Verification items for the finished model (mm, model axes). A direction names the side the tool comes from. Give positions to 0.01 mm unless a question says otherwise; leave off trailing zeros. Loops run counter-clockwise (first coordinate to the right, second up) from the corner with the lowest first, then second, coordinate; pieces in that order, holes last. Notation, with made-up numbers: (-28, 83.25) - (-15, 83.25) arc R21 ccw to (-15, 96.25) - close; hole circle Ø3 at (32, 19.25). An arc over 180 degrees is marked (long way). Answer in a Markdown table with one row per item.
```python
from build123d import *

# Parameters (mm, degrees)
SKETCH1_R               = 3.175
BOSS_EXTRUDE1_DEPTH     = 111.76
SKETCH2_R               = 2.667
BOSS_EXTRUDE2_DEPTH     = 0.762
SKETCH3_R               = 3.175
BOSS_EXTRUDE3_DEPTH     = 1.27
FILLET1_R               = 0.254
CUT_EXTRUDE1_DEPTH      = 114.880553719
CUT_EXTRUDE1_DEPTH_BACK = 114.880553719
SKETCH4_R               = 1.143


with BuildPart() as part:
    # Sketch1 → Boss-Extrude1 (new body)
    with BuildSketch(Plane(origin=(0, 0, 0), x_dir=(0, 0, -1), z_dir=(1, 0, 0))):
        Circle(SKETCH1_R)
    extrude(amount=-BOSS_EXTRUDE1_DEPTH)

    # Sketch2 → Boss-Extrude2 (add)
    with BuildSketch(Plane.ZY.offset(111.76)):
        with Locations(Location((0, 0, 0), (0, 0, 180))):
            Circle(SKETCH2_R)
    extrude(amount=BOSS_EXTRUDE2_DEPTH)

    # Sketch3 → Boss-Extrude3 (add)
    with BuildSketch(Plane.ZY.offset(112.522)):
        with Locations(Location((0, 0, 0), (0, 0, 180))):
            Circle(SKETCH3_R)
    extrude(amount=BOSS_EXTRUDE3_DEPTH)

    # Fillet1
    fillet1_edges = [part.edges().sort_by_distance(p)[0] for p in [
        (-113.792, 0, 3.175),
    ]]
    fillet(fillet1_edges, radius=FILLET1_R)

    # Sketch4 → Cut-Extrude1 (cut, two sides: drawn at the far end of the back side and taken through both)
    with BuildSketch(Plane.XY.offset(-CUT_EXTRUDE1_DEPTH_BACK)):
        with Locations((-60.452, 0)):
            Circle(SKETCH4_R)
        with Locations((-19.05, 0)):
            Circle(SKETCH4_R)
    extrude(amount=CUT_EXTRUDE1_DEPTH + CUT_EXTRUDE1_DEPTH_BACK, mode=Mode.SUBTRACT)


solid = part.part
```
Q1. Sectioned sample at B-B (z = -0.5). Give the number of separate pieces and of enclosed holes in the cut face, and give its area (3 significant figures).
Completed:
| item | result |
|---|---|
| separate pieces | 1 |
| enclosed holes | 2 |
| area | 705 mm^2 |
Q2. Draft check along X on faces 1 (the face through (-61.594, 0.05, -0.044)), 2 (the face through (-113, 2.8, -1.5)), 3 (the face through (0, 0, 0)), 4 (the face through (-113.792, 0, 0)). Enter one of: +X half, -X half, draft (parallel to the pull), parting line (faces both ways), or undercut.
Completed:
| item | result |
|---|---|
| face 1 | undercut |
| face 2 | draft |
| face 3 | +X half |
| face 4 | -X half |
Q3. Tool access check on faces 5 (the face through (-112.136, 2.366, -1.231)), 6 (the face through (-55.1, -3.1, 0.69)). Record the directions out of +Z, -Z, +X, -X, +Y, -Y that give a thin tool (end or side, any length) a straight path to the whole face; none if there is none.
Completed:
| item | result |
|---|---|
| face 5 | none |
| face 6 | +X, -X |
Q4. Sectioned sample at A-A (y = 0). Record the cut outline in (x, z) (3 decimals).
Completed:
| item | result |
|---|---|
| outline | (-113.792, -2.921) arc R0.254 ccw to (-113.538, -3.175) - (-112.522, -3.175) - (-112.522, -2.667) - (-111.76, -2.667) - (-111.76, -3.175) - (-61.595, -3.175) - (-61.595, 3.175) - (-111.76, 3.175) - (-111.76, 2.667) - (-112.522, 2.667) - (-112.522, 3.175) - (-113.538, 3.175) arc R0.254 ccw to (-113.792, 2.921) - close; (-59.309, -3.175) - (-20.193, -3.175) - (-20.193, 3.175) - (-59.309, 3.175) - close; (-17.907, -3.175) - (0, -3.175) - (0, 3.175) - (-17.907, 3.175) - close |
Q5. Thickness scan on line 1 (X direction, y = 0, z = -1.5) (3 decimals); line 2 (Y direction, x = -19.05, z = -0.25); line 3 (Y direction, x = -19.05, z = 1.25). Record the ranges inside material, lowest first.
Completed:
| item | result |
|---|---|
| line 1 | -113.792 to -61.595, -59.309 to -20.193, -17.907 to 0 |
| line 2 | -3.17 to -1.14, 1.14 to 3.17 |
| line 3 | -2.92 to -1.14, 1.14 to 2.92 |
Q6. Go/stop test with a flat-tipped pin: P1, Ø1, axis at x = -36.5, y = -1.5, coming from the +Z side. Record where the tip stops, or that it passes through.
Completed:
| item | result |
|---|---|
| P1 | z = 3.01 |
Q7. Sectioned sample at C-C (x = -19.05). Record the cut outline in (y, z) (3 decimals).
Completed:
| item | result |
|---|---|
| outline | (-1.143, -2.962) - (-1.143, 2.962) arc R3.175 ccw to start; (1.143, -2.962) arc R3.175 ccw to (1.143, 2.962) - close |
